For this review, take the finished solid that the model builds, in its own axes (mm). A direction names the side the tool comes from. Round coordinates to 2 decimals unless told otherwise and drop trailing zeros. Write each loop counter-clockwise with the first axis right and the second up, starting at its lowest first coordinate (ties: lowest second). Pieces come first, ordered by that corner, then holes.
from build123d import *

# Parameters (mm, degrees)
IZIM1_R                              = 9.5
IZIM1_R_2                            = 4
IZIM1_W                              = 70
IZIM1_H                              = 70
Y_KSEKLIK_EKSTR_ZYON1_DEPTH          = 12
Y_KSEKLIK_EKSTR_ZYON2_DEPTH          = 12
KES_EKSTR_ZYON1_START                = -12
KES_EKSTR_ZYON1_DEPTH                = 12
IZIM6_R                              = 4
KES_EKSTR_ZYON4_DEPTH                = 20
M5_HELISARMAL_I_IN_Z_VANA_MATKAB_1_D = 5.2
IZIM9_R                              = 4.1
KES_EKSTR_ZYON5_DEPTH                = 50


with BuildPart() as part:
    # Çizim1 → Yükseklik-Ekstrüzyon1 (new body)
    with BuildSketch(Plane(origin=(0, 0, 0), x_dir=(1, 0, 0), z_dir=(0, 1, 0))):
        with BuildLine():
            ThreePointArc((19.545454545, 40.340909091), (-30.454545455, 90.340909091), (-80.454545455, 40.340909091))
            ThreePointArc((-80.454545455, 40.340909091), (-130.454545455, -9.659090909), (-80.454545455, -59.659090909))
            ThreePointArc((-80.454545455, -59.659090909), (-30.454545455, -109.659090909), (19.545454545, -59.659090909))
            ThreePointArc((19.545454545, -59.659090909), (69.545454545, -9.659090909), (19.545454545, 40.340909091))
        make_face()
        with Locations(Location((-30.454545455, -94.659090909, 0), (0, 0, 270))):
            Circle(IZIM1_R, mode=Mode.SUBTRACT)
        with Locations(Location((-30.454545455, 75.340909091, 0), (0, 0, 270))):
            Circle(IZIM1_R, mode=Mode.SUBTRACT)
        with Locations(Location((54.545454545, -9.659090909, 0), (0, 0, 270))):
            Circle(IZIM1_R_2, mode=Mode.SUBTRACT)
        with Locations(Location((-115.454545455, -9.659090909, 0), (0, 0, 270))):
            Circle(IZIM1_R_2, mode=Mode.SUBTRACT)
        with Locations((-30.454545455, -9.659090909)):
            Rectangle(IZIM1_W, IZIM1_H, mode=Mode.SUBTRACT)
    extrude(amount=Y_KSEKLIK_EKSTR_ZYON1_DEPTH)

    # Çizim2 → Yükseklik-Ekstrüzyon2 (add)
    with BuildSketch(Plane(origin=(0, 12, 0), x_dir=(1, 0, 0), z_dir=(0, 1, 0))):
        with BuildLine():
            ThreePointArc((19.545454545, 40.340909091), (-30.454545455, 90.340909091), (-80.454545455, 40.340909091))
            ThreePointArc((-80.454545455, 40.340909091), (-130.454545455, -9.659090909), (-80.454545455, -59.659090909))
            ThreePointArc((-80.454545455, -59.659090909), (-30.454545455, -109.659090909), (19.545454545, -59.659090909))
            ThreePointArc((19.545454545, -59.659090909), (69.545454545, -9.659090909), (19.545454545, 40.340909091))
        make_face()
    extrude(amount=Y_KSEKLIK_EKSTR_ZYON2_DEPTH)

    # Çizim3 → Kes-Ekstrüzyon1 (cut)
    with BuildSketch(Plane(origin=(0, 24, 0), x_dir=(1, 0, 0), z_dir=(0, 1, 0)).offset(KES_EKSTR_ZYON1_START)):
        with BuildLine():
            Line((-30.454545455, -8.628204493), (-30.454545455, -17.402914961))
            Line((-30.454545455, -17.402914961), (23.509344434, 40.183537201))
            ThreePointArc((23.509344434, 40.183537201), (21.528960845, 40.301550628), (19.545454545, 40.340909091))
            ThreePointArc((19.545454545, 40.340909091), (19.501280543, 42.442206057), (19.368836588, 44.539790114))
            Line((19.368836588, 44.539790114), (-30.454545455, -8.628204493))
        make_face()
    extrude(amount=KES_EKSTR_ZYON1_DEPTH, mode=Mode.SUBTRACT)

    # Çizim6 → Kes-Ekstrüzyon4 (cut)
    with BuildSketch(Plane.XZ):
        with Locations(Location((-115.454545455, 9.659090909, 0), (0, 0, 270))):
            Circle(IZIM6_R)
        with Locations(Location((54.545454545, 9.659090909, 0), (0, 0, 270))):
            Circle(IZIM6_R)
    extrude(amount=-KES_EKSTR_ZYON4_DEPTH, mode=Mode.SUBTRACT)

    # M5 Helisarmal için Zıvana matkabı1 (through all)
    with Locations(Plane(origin=(-80.454545455, 0, 9.659090909), x_dir=(0, 0, -1), z_dir=(0, -1, 0))):
        with Locations((0, 0), (-50, 50), (0, 100), (50, 50)):
            Hole(M5_HELISARMAL_I_IN_Z_VANA_MATKAB_1_D / 2)

    # Çizim9 → Kes-Ekstrüzyon5 (cut)
    with BuildSketch(Plane.XZ):
        with Locations(Location((-30.454545455, 94.659090909, 0), (0, 0, 90))):
            Circle(IZIM9_R)
        with Locations(Location((-30.454545455, -75.340909091, 0), (0, 0, 90))):
            Circle(IZIM9_R)
    extrude(amount=-KES_EKSTR_ZYON5_DEPTH, mode=Mode.SUBTRACT)


solid = part.part
(1) We need section A-A, the plane y = 5.5. State how many separate pieces and enclosed holes the cut face has, and give its area (3 significant figures).
Geometry check:
separate pieces: 1
enclosed holes: 9
area: 20,100 mm2
(2) For faces 5 (the face through (-27.877, 12.168, -40.679)), 6 (the face through (-34.093, 5.916, -66.565)), list the 3-axis set-ups (+Z, -Z, +X, -X, +Y, -Y) from which the entire face can be reached by the end or side of a thin tool; tool diameter is ignored.
Geometry check:
face 5: +Y, -Y
face 6: -Y
(3) Mouldability with a two-part tool opening along Z and no side actions: class faces 1 (the face through (4.545, 6, 10)), 2 (the face through (-32, 24, 8)), 3 (the face through (-115, 20, 10)), 4 (the face through (69.533, 11.832, 10.759)) as pulls with the +Z half, pulls with the -Z half, needs draft (parallel to the pull), parting line crosses it, or undercut.
Geometry check:
face 1: undercut
face 2: needs draft
face 3: undercut
face 4: parting line crosses it
(4) We need section C-C, the plane z = 21.5. Give the boundary of the cut face in (x, y).
Geometry check:
outline: (-129.03, 0) - (-65.45, 0) - (-65.45, 12) - (4.55, 12) - (4.55, 0) - (68.12, 0) - (68.12, 24) - (-129.03, 24) - close
(5) We need section B-B, the plane z = -2.5. Give the boundary of the cut face in (x, y).
Geometry check:
outline: (-128.95, 0) - (-65.45, 0) - (-65.45, 12) - (-20.03, 12) - (-20.03, 24) - (-128.95, 24) - close; (-11.8, 12) - (4.55, 12) - (4.55, 0) - (68.04, 0) - (68.04, 24) - (-11.8, 24) - close
(6) We need section D-D, the plane x = -72. Give the boundary of the cut face in (y, z), and give its area (3 significant figures).
Geometry check:
outline: (0, -68.16) - (24, -68.16) - (24, 87.48) - (0, 87.48) - close
area: 3,740 mm2
(7) For line 1 along Z through (x, y) = (-30.5, 14.5); line 2 along Z through (x, y) = (20, 11.75); line 3 along Z through (x, y) = (-56.5, 5.5), list the stretches that pass through material, from the lowest coordinate up.
Geometry check:
line 1: z = -90.34 to -79.44, -71.24 to -42.94, -37.74 to 57.06, 62.26 to 90.56, 98.76 to 109.66
line 2: z = -40.34 to 7.1, 12.22 to 59.66
line 3: z = -83.02 to -25.34, 44.66 to 102.34
(8) For pin 1 Ø17 at (x, z) = (-30.45, 94.66) entering from -Y; pin 2 Ø8 at (y, z) = (20, -58.5) entering from +X; pin 3 Ø3 at (x, z) = (-30.45, -40.34) entering from -Y (1 decimal); pin 4 Ø13 at (x, y) = (-33.5, 4) entering from -Z, all flat-tipped, find the tip position at first contact; note any pin that passes through.
Geometry check:
pin 1: stops at y = 12
pin 2: stops at x = 17.5
pin 3: passes through
pin 4: stops at z = -90.34
